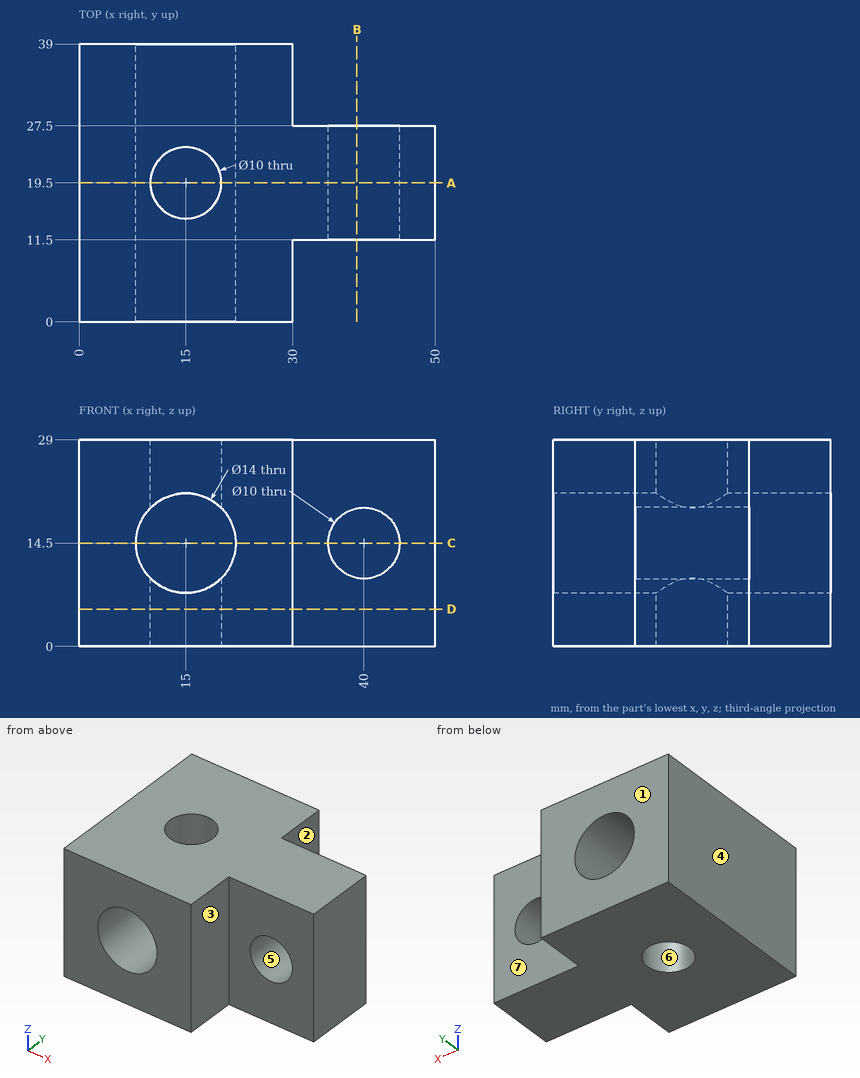
Design review of the part shown in the three views and the two pictorial views. Dimensions are in mm from the part's minimum x, y and z. A direction names the side the tool comes from. Give positions to 0.01 mm unless a question says otherwise; leave off trailing zeros. Loops run counter-clockwise (first coordinate to the right, second up) from the corner with the lowest first, then second, coordinate; pieces in that order, holes last. Notation, with made-up numbers: M 62.5,31 L 82.5,31 A25 cw 82.5,56 Z; hole C -23.5,27.25 d7. An arc over 180 degrees is marked long. Put each result on its own line as item: value. Start each with the question number.
(1) Add section C-C, the plane z = 14.5. Write out the cut boundary in (x, y).
(2) The part is to be moulded in two halves that separate along X. For the marked faces 4, 5, 6 and 7, say which applies: +X half, -X half, draft (parallel to the pull), parting line (faces both ways), or undercut.
(3) Wall thickness on L1, parallel to X at y = 12.5, z = 14.5; L2, parallel to Y at x = 15, z = 3.5; L3, parallel to Z at x = 10, y = 4: over which ranges is each line inside the solid? List them lowest first.
(4) For pin 1 (10 mm diameter, centred on x = 36.5, z = 9, fed in from -Y); pin 2 (1.5 mm diameter, centred on x = 34.5, z = 10.5, fed in from +Y); pin 3 (6 mm diameter, centred on y = 6.5, z = 14.5, fed in from +X); pin 4 (2 mm diameter, centred on x = 35.5, y = 9, fed in from -Z), all flat-tipped, find the tip position at first contact; note any pin that passes through.
(5) Machinability: for the marked faces 1, 2 and 3, which of the approach directions +Z, -Z, +X, -X, +Y, -Y give a long, thin tool a straight path to every point of the face, cutting with its end or side? Answer none if there is none.
(6) Add section A-A, the plane y = 19.5. Write out the cut boundary in (x, z), then the cut area to 3 significant figures.
(7) Add section D-D, the plane z = 5.25. Write out the cut boundary in (x, y).
(8) Add section B-B, the plane x = 39. Write out the cut boundary in (y, z).
Result:
1. outline: M 0,0 L 8,0 L 8,39 L 0,39 Z; M 22,0 L 30,0 L 30,11.5 L 35,11.5 L 35,27.5 L 30,27.5 L 30,39 L 22,39 Z; M 45,11.5 L 50,11.5 L 50,27.5 L 45,27.5 Z
2. face 4: -X half
2. face 5: undercut
2. face 6: undercut
2. face 7: draft
3. L1: x = 0 to 8, 22 to 35, 45 to 50
3. L2: y = 0 to 14.5, 24.5 to 39
3. L3: z = 0 to 9.6, 19.4 to 29
4. pin 1: stops at y = 11.5
4. pin 2: stops at y = 27.5
4. pin 3: stops at x = 30
4. pin 4: passes through
5. face 1: +Z, -Z, +X, -X, +Y
5. face 2: +Z, -Z, +X, +Y
5. face 3: +Z, -Z, +X, -Y
6. outline: M 0,0 L 10,0 L 10,9.6 A7 cw 10,19.4 L 10,29 L 0,29 Z; M 20,0 L 50,0 L 50,29 L 20,29 L 20,19.4 A7 cw 20,9.6 Z; hole C 40,14.5 d10
6. area: 1,050 mm^2
7. outline: M 0,0 L 30,0 L 30,11.5 L 50,11.5 L 50,27.5 L 30,27.5 L 30,39 L 0,39 Z; hole C 15,19.5 d10
8. outline: M 11.5,0 L 27.5,0 L 27.5,9.6 L 11.5,9.6 Z; M 11.5,19.4 L 27.5,19.4 L 27.5,29 L 11.5,29 Z
